For this review, use the dimensioned drawing (mm, ordinates from the lowest corner) and the shaded views. A direction names the side the tool comes from. Round coordinates to 2 decimals unless told otherwise and drop trailing zeros. Loops run counter-clockwise (first coordinate to the right, second up) from the corner with the lowest first, then second, coordinate; pieces in that order, holes last. Notation, with made-up numbers: M 62.5,-27 L 74.5,-27 A24 ccw 74.5,7 Z; hole C 2.25,3 d7. An arc over 180 degrees is marked long. Answer as a JSON object with one key per item and string values. Group by question number.
Item 1: Consider section B-B (x = 13.5). Give the boundary of the cut face in (y, z), and give its area (3 significant figures).
Item 2: Tool access review of the marked faces 1, 2 and 3: name each direction out of +Z, -Z, +X, -X, +Y, -Y from which nothing blocks a thin tool from reaching the whole face with its end or side.
Item 3: Consider section C-C (y = 17.25). Give the boundary of the cut face in (x, z).
Item 4: Insertion check: P1, Ø6, axis at x = 21.5, y = 20.5, coming from the +Z side; P2, Ø4, axis at x = 14, z = 22.5, coming from the +Y side; P3, Ø4, axis at x = 15, y = 21.5, coming from the -Z side. Each pin has a flat end and moves straight along its axis. Give the tip position at first contact, or say it passes through.
Item 5: To check wall thickness, follow line 1 (Y direction, x = 15.75, z = 7.25); line 2 (Y direction, x = 7.5, z = 8.5); line 3 (X direction, y = 18, z = 18). State the ranges of each line that lie inside material, in increasing order.
Item 6: Consider section A-A (z = 13.5). Give the boundary of the cut face in (x, y).
Item 7: Consider section D-D (y = 2.25). Give the boundary of the cut face in (x, z), and give its area (3 significant figures).
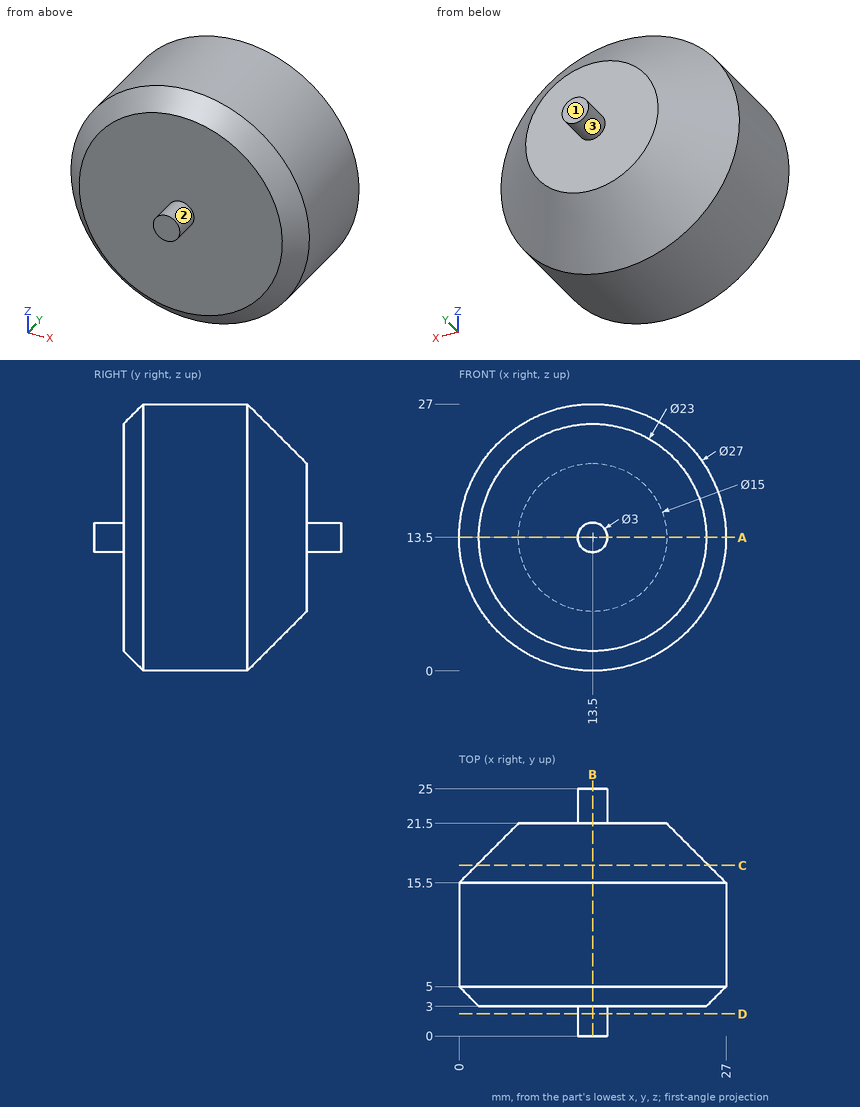
Geometry results:
{
 "1": {"outline": "M 0,12 L 3,12 L 3,2 L 5,0 L 15.5,0 L 21.5,6 L 21.5,12 L 25,12 L 25,15 L 21.5,15 L 21.5,21 L 15.5,27 L 5,27 L 3,25 L 3,15 L 0,15 Z", "area": "479 mm^2"},
 "2": {"face 1": "+Z, -Z, +X, -X, +Y", "face 2": "-Y", "face 3": "+Y"},
 "3": {"outline": "C 13.5,13.5 d23.5"},
 "4": {"P1": "stops at z = 22.5", "P2": "stops at y = 21.5", "P3": "stops at z = 4.1"},
 "5": {"line 1": "y = 3 to 21.5", "line 2": "y = 3 to 21.19", "line 3": "x = 3.46 to 23.54"},
 "6": {"outline": "M 0,5 L 2,3 L 12,3 L 12,0 L 15,0 L 15,3 L 25,3 L 27,5 L 27,15.5 L 21,21.5 L 15,21.5 L 15,25 L 12,25 L 12,21.5 L 6,21.5 L 0,15.5 Z"},
 "7": {"outline": "C 13.5,13.5 d3", "area": "7.07 mm^2"}
}
